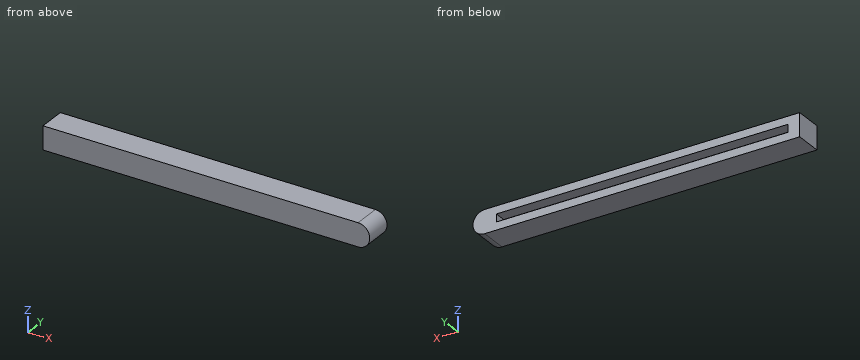
```python
from build123d import *

# Parameters (mm, degrees)
SKETCH_1_R          = 1.5
EXTRUDE_1_DEPTH     = 3.5
SKETCH_2_W          = 37.5
SKETCH_2_H          = 1
CUT_EXTRUDE_1_DEPTH = 1.5


with BuildPart() as part:
    # 草图1 → 凸台-拉伸1 (new body)
    with BuildSketch(Plane(origin=(0, 0, 0), x_dir=(1, 0, 0), z_dir=(0, 1, 0))):
        with BuildLine():
            Line((40.5, 0), (0, 0))
            Line((0, 0), (0, -3))
            Line((0, -3), (40.5, -3))
            ThreePointArc((40.5, -3), (39, -1.5), (40.5, 0))
        make_face()
        with Locations((40.5, -1.5)):
            Circle(SKETCH_1_R)
    extrude(amount=EXTRUDE_1_DEPTH)

    # 草图2 → 切除-拉伸1 (cut)
    with BuildSketch(Plane(origin=(0, 3.5, 0), x_dir=(1, 0, 0), z_dir=(0, 1, 0))):
        with Locations((20.25, -1.5)):
            Rectangle(SKETCH_2_W, SKETCH_2_H)
    extrude(amount=-CUT_EXTRUDE_1_DEPTH, mode=Mode.SUBTRACT)


solid = part.part
```
Part model, mm, in its own coordinate system. Round coordinates to 2 decimals unless told otherwise and drop trailing zeros. Write each loop counter-clockwise with the first axis right and the second up, starting at its lowest first coordinate (ties: lowest second). Pieces come first, ordered by that corner, then holes.
Item 1: Probe L1, parallel to Z at x = 10, y = 3.4; L2, parallel to X at y = 2.2, z = 1.6; L3, parallel to Y at x = 11.5, z = 1.1. List the from-to ranges inside material, lowest first.
Results:
L1: z = 0 to 1, 2 to 3
L2: x = 0 to 1.5, 39 to 42
L3: y = 0 to 2
Item 2: Cut at B-B, the plane z = 1.5. Give the cut face in (x, y), plus the area to 4 significant figures.
Results:
outline: (0, 0) - (42, 0) - (42, 3.5) - (39, 3.5) - (39, 2) - (1.5, 2) - (1.5, 3.5) - (0, 3.5) - close
area: 90.75 mm2
Item 3: Cut at C-C, the plane x = 37. Give the cut face in (y, z).
Results:
outline: (0, 0) - (3.5, 0) - (3.5, 1) - (2, 1) - (2, 2) - (3.5, 2) - (3.5, 3) - (0, 3) - close
Item 4: Cut at A-A, the plane y = 2.4. Give the cut face in (x, z), plus the area to 3 significant figures.
Results:
outline: (0, 0) - (40.5, 0) arc R1.5 ccw to (40.5, 3) - (0, 3) - close; hole (1.5, 1) - (39, 1) - (39, 2) - (1.5, 2) - close
area: 87.5 mm2
Item 5: Drop a flat-ended pin along its axis: pin 1 Ø0.5 at (x, z) = (25.5, 1.5) entering from +Y. Give the stop position or say it passes through.
Results:
pin 1: stops at y = 2
